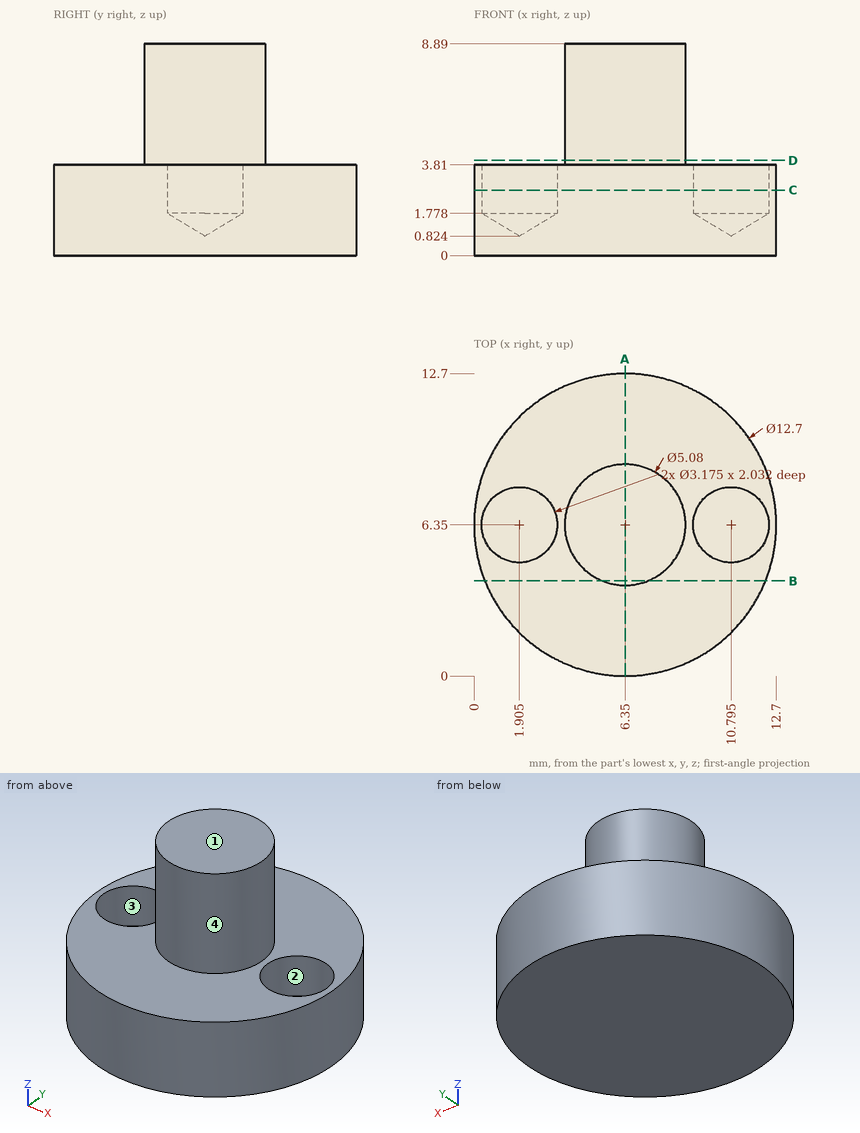
Geometry check sheet. Reference: drawing and pictorial views, mm from the part's lowest x, y, z. Coordinates: 2 decimals unless noted, no trailing zeros. Order: outer loops, then holes, each group sorted by start corner. A loop starts at its lowest first (then second) coordinate and runs counter-clockwise, first axis right, second up. Notation, with made-up numbers: M -14,-34 L 31,-34 A31 ccw 31,1 Z; hole C 62,11 d4. An arc over 180 degrees is marked long. Return JSON: item names as keys, results as strings.
1) Cross-section at D-D, the plane z = 4. Record the boundary of the cut face in (x, y), and give its area (3 significant figures).
Answer list:
{"outline": "C 6.35,6.35 d5.08", "area": "20.3 mm2"}
2) Release check for a two-part mould opening along X. For the marked faces 1, 2, 3 and 4 record: +X half, -X half, draft (parallel to the pull), parting line (faces both ways), or undercut.
Answer list:
{"face 1": "draft", "face 2": "undercut", "face 3": "undercut", "face 4": "parting line"}
3) Thickness scan on L1, parallel to X at y = 7.5, z = 2.75 (1 decimal); L2, parallel to Z at x = 11.25, y = 10; L3, parallel to Y at x = 10.5, z = 2. Record the ranges inside material, lowest first. Write a range as [from, to].
Answer list:
{"L1": "[0.1, 0.8], [3, 9.7], [11.9, 12.6]", "L2": "[0, 3.81]", "L3": "[1.54, 4.79], [7.91, 11.16]"}
4) Cross-section at A-A, the plane x = 6.35. Record the boundary of the cut face in (y, z), and give its area (3 significant figures).
Answer list:
{"outline": "M 0,0 L 12.7,0 L 12.7,3.81 L 8.89,3.81 L 8.89,8.89 L 3.81,8.89 L 3.81,3.81 L 0,3.81 Z", "area": "74.2 mm2"}
5) Gauge pin test, flat ends, axial feed: pin 1 (4 mm diameter, centred on x = 11.5, z = 4, fed in from -Y); pin 2 (4 mm diameter, centred on x = 8, z = 5.5, fed in from -Y); pin 3 (1.9 mm diameter, centred on x = 1.905, y = 6.35, fed in from +Z) (3 decimals). Record the tip position at first contact, or that the pin passes through.
Answer list:
{"pin 1": "y = 0.84", "pin 2": "y = 0.03", "pin 3": "z = 1.395"}
6) Cross-section at B-B, the plane y = 4. Record the boundary of the cut face in (x, z).
Answer list:
{"outline": "M 0.45,0 L 12.25,0 L 12.25,3.81 L 7.31,3.81 L 7.31,8.89 L 5.39,8.89 L 5.39,3.81 L 0.45,3.81 Z"}
7) Cross-section at C-C, the plane z = 2.75. Count the separate pieces of the cut face and the enclosed holes in it, and give its area (3 significant figures).
Answer list:
{"separate pieces": "1", "enclosed holes": "2", "area": "111 mm2"}
